from build123d import *

# Parameters (mm, degrees)
F0_W        = 105
F0_H        = 45
F0_R        = 1.875
F0_R_2      = 13
F1_DEPTH    = 5
F2_W        = 115
F2_H        = 55
F2_W_2      = 105
F2_H_2      = 4.9815587699
F3_DEPTH    = 80
F4_W        = 2.5
F4_H        = 10
F5_DEPTH    = 115.001
F6_R        = 2.5
F7_T1_DEPTH = 92.5
F7_T4_ANGLE = 90
F7_T6_ANGLE = 90
F8_W        = 10.5
F8_H        = 27.5
F9_DEPTH    = 5
F10_W       = 10
F10_H       = 15
F11_DEPTH   = 5.001
F12_R       = 1.5


# Not quite as in the source:
# - a fillet or chamfer that OpenCascade refuses, or shapes differently, is made with other operations: its cross-section is extruded or revolved along the edge and cut away or added


with BuildPart() as f1:
    # F0 (on Front) → F1 (new body)
    with BuildSketch(Plane.XZ):
        Rectangle(F0_W, F0_H)
        with Locations((-43, -13)):
            Circle(F0_R, mode=Mode.SUBTRACT)
        with Locations((43, -13)):
            Circle(F0_R, mode=Mode.SUBTRACT)
        with Locations((-22, 0)):
            Circle(F0_R_2, mode=Mode.SUBTRACT)
        with Locations((-43, 13)):
            Circle(F0_R, mode=Mode.SUBTRACT)
        with Locations((22, 0)):
            Circle(F0_R_2, mode=Mode.SUBTRACT)
        with Locations((43, 13)):
            Circle(F0_R, mode=Mode.SUBTRACT)
    extrude(amount=F1_DEPTH)

    # F2 (on face) → F3 (join)
    with BuildSketch(Plane.XZ.offset(5)):
        Rectangle(F2_W, F2_H)
        Polygon((-52.5, -22.5), (-52.5, 22.5), (52.5, 22.5), (52.5, -22.5), (52.5, -27.4815587699), (-52.5, -27.4815587699), align=None, mode=Mode.SUBTRACT)
        with Locations((0, -24.990779385)):
            Rectangle(F2_W_2, F2_H_2)
    extrude(amount=-F3_DEPTH)

    # F4 (on face) → F5 (cut, through all)
    with BuildSketch(Plane.YZ.offset(57.5)):
        with Locations((26.25, -22.5)):
            Rectangle(F4_W, F4_H)
    extrude(amount=-F5_DEPTH, mode=Mode.SUBTRACT)

    # F6
    f6_edges = [f1.edges().sort_by_distance(p)[0] for p in [
        (0, -5, 27.5),
        (-57.5, -5, 0),
        (0, -5, -27.5),
        (57.5, -5, 0),
    ]]
    fillet(f6_edges, radius=F6_R)

    # F7: fillet of radius 5 on 2 edges, made by hand

    # F7_s2 → F7_t1 (cut)
    with BuildSketch(Plane.XZ.offset(-87.5)):
        with BuildLine():
            ThreePointArc((-52.5, 27.5), (-56.0355339059, 26.0355339059), (-57.5, 22.5))
            Line((-57.5, 22.5), (-57.5, 27.5))
            Line((-57.5, 27.5), (-52.5, 27.5))
        make_face()
        with BuildLine():
            ThreePointArc((52.5, 27.5), (56.0355339059, 26.0355339059), (57.5, 22.5))
            Line((57.5, 22.5), (57.5, 27.5))
            Line((57.5, 27.5), (52.5, 27.5))
        make_face()
    extrude(amount=F7_T1_DEPTH, mode=Mode.SUBTRACT)

    # F7_s3 → F7_t4 (revolve, cut)
    with BuildSketch(Plane.XY.offset(22.5)):
        with BuildLine():
            ThreePointArc((55, -5), (56.767766953, -4.267766953), (57.5, -2.5))
            Line((57.5, -2.5), (57.5, -5))
            Line((57.5, -5), (55, -5))
        make_face()
    revolve(axis=Axis((52.5, -5, 22.5), (0, -1, 0)), revolution_arc=F7_T4_ANGLE, mode=Mode.SUBTRACT)

    # F7_s5 → F7_t6 (revolve, cut)
    with BuildSketch(Plane.YZ.offset(-52.5)):
        with BuildLine():
            ThreePointArc((-5, 25), (-4.267766953, 26.767766953), (-2.5, 27.5))
            Line((-2.5, 27.5), (-5, 27.5))
            Line((-5, 27.5), (-5, 25))
        make_face()
    revolve(axis=Axis((-52.5, -5, 22.5), (0, -1, 0)), revolution_arc=F7_T6_ANGLE, mode=Mode.SUBTRACT)

    # F8 (on face) → F9 (cut, through all)
    with BuildSketch(Plane.XY.offset(27.5)):
        with Locations((45.25, 58.25)):
            Rectangle(F8_W, F8_H)
    extrude(amount=-F9_DEPTH, mode=Mode.SUBTRACT)

    # F10 (on face) → F11 (cut, through all)
    with BuildSketch(Plane(origin=(52.5, 0, 0), x_dir=(0, -1, 0), z_dir=(-1, 0, 0))):
        with Locations((-70, -15)):
            Rectangle(F10_W, F10_H)
    extrude(amount=-F11_DEPTH, mode=Mode.SUBTRACT)

    # F12
    f12_edges = [f1.edges().sort_by_distance(p)[0] for p in [
        (0, 0, -22.5),
        (52.5, 0, 0),
        (0, 0, 22.5),
        (-52.5, 0, 0),
        (-52.5, 37.5, 22.5),
        (52.5, 37.5, 22.5),
        (52.5, 12.5, -22.5),
        (52.5, 46.25, -22.5),
        (-52.5, 12.5, -22.5),
        (-52.5, 51.25, -22.5),
    ]]
    fillet(f12_edges, radius=F12_R)


solid = f1.part
Could you check a few things on this model? Use its own coordinates, in mm. A direction names the side the tool comes from. Coordinates: 2 decimals unless noted, no trailing zeros. Order: outer loops, then holes, each group sorted by start corner. A loop starts at its lowest first (then second) coordinate and runs counter-clockwise, first axis right, second up. Notation, with made-up numbers: (48, -23) -> (88, -23) arc R13 cw to (88, -8) -> close; hole circle Ø9 at (64, -6.75). An arc over 180 degrees is marked (long way). One line per item, written item: value. Start each with the question number.
1) Imagine slicing it at D-D on z = 7. List the corners of the cut face in (x, y) for me, plus the area to 3 significant figures.
2) I'm going to push flat-ended pins straight in: pin 1 (6 mm diameter, centred on x = 43, z = 13, fed in from +Y); pin 2 (4 mm diameter, centred on y = 55.5, z = 26, fed in from +X); pin 3 (5 mm diameter, centred on x = 54, z = -17.5, fed in from +Y); pin 4 (3.5 mm diameter, centred on x = -43, z = 13, fed in from +Y). Where does each tip first touch, or does it pass through?
3) If I drill on L1, parallel to Z at x = -43, y = -2 (3 decimals); L2, parallel to X at y = 34.5, z = -21; L3, parallel to Y at x = -52, z = -23.5, over which ranges is the centre line in solid material (lowest first)? Write a range as [from, to].
4) We'd pull the mould along Z, two halves only. Please class faces 1 (the flat face through (50.5, 58, 25)), 2 (the cylindrical face through (-9.6, -2.5, 3.9)), 3 (the cylindrical face through (1, -4, 27)): +Z half, -Z half, draft (parallel to the pull), parting line (faces both ways), or undercut.
5) Imagine slicing it at A-A on x = -22. List the corners of the cut face in (y, z) for me, plus the area to 3 significant figures.
6) Imagine slicing it at C-C on y = 30. List the corners of the cut face in (x, z) for me, plus the area to 3 significant figures.
7) Imagine slicing it at B-B on x = 43. List the corners of the cut face in (y, z) for me (3 decimals), plus the area to 3 significant figures.
8) Which directions (+Z, -Z, +X, -X, +Y, -Y) give clear straight access to the entire face, cutting with the end or side of a thin tool? Please do faces 4 (the flat face through (1, 25, -25)), 5 (the flat face through (-1, 13, -22.5)), 6 (the flat face through (45, 72, 25)).
Answer list:
1. outline: (-57.5, -2.5) arc R2.5 ccw to (-55, -5) -> (-32.95, -5) -> (-32.95, 0) -> (-51, 0) arc R1.5 cw to (-52.5, 1.5) -> (-52.5, 75) -> (-57.5, 75) -> close; (-11.05, -5) -> (11.05, -5) -> (11.05, 0) -> (-11.05, 0) -> close; (32.95, -5) -> (55, -5) arc R2.5 ccw to (57.5, -2.5) -> (57.5, 75) -> (52.5, 75) -> (52.5, 1.5) arc R1.5 cw to (51, 0) -> (32.95, 0) -> close
1. area: 1,100 mm2
2. pin 1: stops at y = 0
2. pin 2: stops at x = 57.27
2. pin 3: stops at y = 65
2. pin 4: passes through
3. L1: z = [-27.5, -14.875], [-11.125, 11.125], [14.875, 27.5]
3. L2: x = [-57.5, -52.5], [52.5, 57.5]
3. L3: y = [-5, 25], [27.5, 75]
4. face 1: draft
4. face 2: undercut
4. face 3: +Z half
5. outline: (-5, -25) arc R2.5 ccw to (-2.5, -27.5) -> (25, -27.5) -> (25, -22.5) -> (1.5, -22.5) arc R1.5 cw to (0, -21) -> (0, -13) -> (-5, -13) -> close; (-5, 13) -> (0, 13) -> (0, 21) arc R1.5 cw to (1.5, 22.5) -> (75, 22.5) -> (75, 27.5) -> (-2.5, 27.5) arc R2.5 ccw to (-5, 25) -> close; (27.5, -27.5) -> (75, -27.5) -> (75, -22.5) -> (27.5, -22.5) -> close
5. area: 881 mm2
6. outline: (-57.5, -27.5) -> (57.5, -27.5) -> (57.5, 22.5) arc R5 ccw to (52.5, 27.5) -> (-52.5, 27.5) arc R5 ccw to (-57.5, 22.5) -> close; hole (-52.5, -21) arc R1.5 ccw to (-51, -22.5) -> (51, -22.5) arc R1.5 ccw to (52.5, -21) -> (52.5, 21) arc R1.5 ccw to (51, 22.5) -> (-51, 22.5) arc R1.5 ccw to (-52.5, 21) -> close
6. area: 1,590 mm2
7. outline: (-5, -25) arc R2.5 ccw to (-2.5, -27.5) -> (25, -27.5) -> (25, -22.5) -> (1.5, -22.5) arc R1.5 cw to (0, -21) -> (0, -14.875) -> (-5, -14.875) -> close; (-5, -11.125) -> (0, -11.125) -> (0, 11.125) -> (-5, 11.125) -> close; (-5, 14.875) -> (0, 14.875) -> (0, 21) arc R1.5 cw to (1.5, 22.5) -> (44.5, 22.5) -> (44.5, 27.5) -> (-2.5, 27.5) arc R2.5 ccw to (-5, 25) -> close; (27.5, -27.5) -> (75, -27.5) -> (75, -22.5) -> (27.5, -22.5) -> close; (72, 22.5) -> (75, 22.5) -> (75, 27.5) -> (72, 27.5) -> close
7. area: 836 mm2
8. face 4: -Z, +X, -X
8. face 5: +Y
8. face 6: +Z
